Here's how the part is built. I have some questions about the finished solid (model axes, mm). A direction names the side the tool comes from. Coordinates: 2 decimals unless noted, no trailing zeros. Write each loop counter-clockwise with the first axis right and the second up, starting at its lowest first coordinate (ties: lowest second). Pieces come first, ordered by that corner, then holes. Notation, with made-up numbers: M -30.5,-10 L -2.5,-10 A13 ccw -2.5,-6 Z; hole C -31.75,19 d10. An arc over 180 degrees is marked long. Use a Markdown table: item, result.
```python
from build123d import *

# Parameters (mm, degrees)
BOSS_EXTRUDE2_DEPTH      = 3.175
SKETCH4_R                = 38.1
CUT_EXTRUDE3_DEPTH       = 92.247975457
CUT_EXTRUDE6_DEPTH       = 92.247975457
BOSS_EXTRUDE3_DEPTH      = 3.175
SKETCH12_R               = 1.143
CUT_EXTRUDE9_DEPTH       = 97.166400707
SKETCH14_R               = 3.175
CUT_EXTRUDE11_DEPTH      = 103.378
CUT_EXTRUDE11_DEPTH_BACK = 116.832157669
SKETCH15_R               = 1.651
CUT_EXTRUDE12_DEPTH      = 75.692
SKETCH17_R               = 1.651
CUT_EXTRUDE14_DEPTH      = 97.79
SKETCH18_R               = 12.192
CUT_EXTRUDE15_DEPTH      = 35.56


with BuildPart() as part:
    # Sketch1 → Boss-Extrude2 (new body)
    with BuildSketch(Plane.XY):
        with BuildLine():
            Line((-60.107370596, 33.02), (-55.027370596, 33.02))
            Line((-55.027370596, 33.02), (-55.027370596, -33.02))
            Line((-55.027370596, -33.02), (-60.107370596, -33.02))
            ThreePointArc((-60.107370596, -33.02), (0, -68.58), (60.107370596, -33.02))
            Line((60.107370596, -33.02), (55.027370596, -33.02))
            Line((55.027370596, -33.02), (55.027370596, 33.02))
            Line((55.027370596, 33.02), (60.107370596, 33.02))
            ThreePointArc((60.107370596, 33.02), (0, 68.58), (-60.107370596, 33.02))
        make_face()
    extrude(amount=BOSS_EXTRUDE2_DEPTH)

    # Sketch4 → Cut-Extrude3 (cut, through all)
    with BuildSketch(Plane(origin=(0, 0, 0), x_dir=(-1, 0, 0), z_dir=(0, 0, -1))):
        with Locations((0, -86.312058398)):
            Circle(SKETCH4_R)
    extrude(amount=-CUT_EXTRUDE3_DEPTH, mode=Mode.SUBTRACT)

    # Sketch5 → Cut-Extrude6 (cut, through all)
    with BuildSketch(Plane(origin=(0, 0, 0), x_dir=(-1, 0, 0), z_dir=(0, 0, -1))):
        with BuildLine():
            ThreePointArc((45.008715274, -51.743907365), (46.779291091, -50.148921474), (48.493383054, -48.493383054))
            Line((48.493383054, -48.493383054), (33.244765274, -33.244765274))
            Line((33.244765274, -33.244765274), (15.050661462, -15.479201839))
            ThreePointArc((15.050661462, -15.479201839), (11.453327097, -13.609958514), (12.680560823, -17.473736785))
            Line((12.680560823, -17.473736785), (29.410338797, -36.145530887))
            Line((29.410338797, -36.145530887), (45.008715274, -51.743907365))
        make_face()
        with BuildLine():
            ThreePointArc((-48.493383054, -48.493383054), (-46.779291091, -50.148921474), (-45.008715274, -51.743907365))
            Line((-45.008715274, -51.743907365), (-29.410338797, -36.145530887))
            Line((-29.410338797, -36.145530887), (-12.680560823, -17.473736785))
            ThreePointArc((-12.680560823, -17.473736785), (-11.453327097, -13.609958514), (-15.050661462, -15.479201839))
            Line((-15.050661462, -15.479201839), (-33.244765274, -33.244765274))
            Line((-33.244765274, -33.244765274), (-48.493383054, -48.493383054))
        make_face()
        with BuildLine():
            Line((-29.410338797, 36.145530887), (-45.008715274, 51.743907365))
            ThreePointArc((-45.008715274, 51.743907365), (-46.779291091, 50.148921474), (-48.493383054, 48.493383054))
            Line((-48.493383054, 48.493383054), (-33.244765274, 33.244765274))
            Line((-33.244765274, 33.244765274), (-15.050661462, 15.479201839))
            ThreePointArc((-15.050661462, 15.479201839), (-11.453327097, 13.609958514), (-12.680560823, 17.473736785))
            Line((-12.680560823, 17.473736785), (-29.410338797, 36.145530887))
        make_face()
        with BuildLine():
            Line((33.244765274, 33.244765274), (48.493383054, 48.493383054))
            ThreePointArc((48.493383054, 48.493383054), (46.779291091, 50.148921474), (45.008715274, 51.743907365))
            Line((45.008715274, 51.743907365), (29.410338797, 36.145530887))
            Line((29.410338797, 36.145530887), (12.680560823, 17.473736785))
            ThreePointArc((12.680560823, 17.473736785), (11.453327097, 13.609958514), (15.050661462, 15.479201839))
            Line((15.050661462, 15.479201839), (33.244765274, 33.244765274))
        make_face()
    extrude(amount=-CUT_EXTRUDE6_DEPTH, mode=Mode.SUBTRACT)

    # Sketch9 → Boss-Extrude3 (add)
    with BuildSketch(Plane(origin=(0, 0, 0), x_dir=(-1, 0, 0), z_dir=(0, 0, -1))):
        with BuildLine():
            Line((12.7, 67.39381574), (0, 75))
            Line((0, 75), (-12.7, 67.39381574))
            ThreePointArc((-12.7, 67.39381574), (0, 68.58), (12.7, 67.39381574))
        make_face()
    extrude(amount=-BOSS_EXTRUDE3_DEPTH)

    # Sketch12 → Cut-Extrude9 (cut, through all)
    with BuildSketch(Plane(origin=(0, 0, 0), x_dir=(-1, 0, 0), z_dir=(0, 0, -1))):
        with Locations((6.731, 62.23)):
            Circle(SKETCH12_R)
        with Locations((-6.731, 62.23)):
            Circle(SKETCH12_R)
    extrude(amount=-CUT_EXTRUDE9_DEPTH, mode=Mode.SUBTRACT)

    # Sketch14 → Cut-Extrude11 (cut, two sides)
    with BuildSketch(Plane(origin=(30.092005081, 4.08352975, 15.875), x_dir=(-1, 0, 0), z_dir=(0, 0, -1))) as cut_extrude11_sk:
        with Locations(Location((-13.087994919, 21.31647025, 0), (0, 0, 180))):
            Circle(SKETCH14_R)
        with Locations(Location((73.272005081, 21.31647025, 0), (0, 0, 180))):
            Circle(SKETCH14_R)
        with Locations(Location((30.092005081, 21.31647025, 0), (0, 0, 180))):
            Circle(SKETCH14_R)
        with Locations(Location((73.272005081, -29.48352975, 0), (0, 0, 180))):
            Circle(SKETCH14_R)
        with Locations(Location((30.092005081, -29.48352975, 0), (0, 0, 180))):
            Circle(SKETCH14_R)
        with Locations(Location((-13.087994919, -29.48352975, 0), (0, 0, 180))):
            Circle(SKETCH14_R)
    extrude(amount=CUT_EXTRUDE11_DEPTH, mode=Mode.SUBTRACT)
    extrude(cut_extrude11_sk.sketch, amount=-CUT_EXTRUDE11_DEPTH_BACK, mode=Mode.SUBTRACT)

    # Sketch15 → Cut-Extrude12 (cut)
    with BuildSketch(Plane(origin=(30.092005081, 4.08352975, -25.527), x_dir=(-1, 0, 0), z_dir=(0, 0, -1))):
        with Locations(Location((63.757223581, 17.50647025, 0), (0, 0, 180))):
            Circle(SKETCH15_R)
        with Locations(Location((63.757223581, -25.67352975, 0), (0, 0, 180))):
            Circle(SKETCH15_R)
        with Locations(Location((-3.552776419, -25.67352975, 0), (0, 0, 180))):
            Circle(SKETCH15_R)
        with Locations(Location((-3.552776419, 17.50647025, 0), (0, 0, 180))):
            Circle(SKETCH15_R)
    extrude(amount=-CUT_EXTRUDE12_DEPTH, mode=Mode.SUBTRACT)

    # Sketch17 → Cut-Extrude14 (cut)
    with BuildSketch(Plane(origin=(30.092005081, 4.08352975, -31.75), x_dir=(-1, 0, 0), z_dir=(0, 0, -1))):
        with Locations(Location((4.154396091, -49.728759131, 0), (0, 0, 180))):
            Circle(SKETCH17_R)
        with Locations(Location((56.02961407, -49.728759131, 0), (0, 0, 180))):
            Circle(SKETCH17_R)
        with Locations(Location((4.154396091, 41.38247025, 0), (0, 0, 180))):
            Circle(SKETCH17_R)
        with Locations(Location((56.02961407, 41.38247025, 0), (0, 0, 180))):
            Circle(SKETCH17_R)
    extrude(amount=-CUT_EXTRUDE14_DEPTH, mode=Mode.SUBTRACT)

    # Sketch18 → Cut-Extrude15 (cut)
    with BuildSketch(Plane(origin=(0, 0, 0), x_dir=(-1, 0, 0), z_dir=(0, 0, -1))):
        with Locations((31.75, 0)):
            Circle(SKETCH18_R)
        with Locations(Location((-31.75, 0, 0), (0, 0, 180))):
            Circle(SKETCH18_R)
    extrude(amount=-CUT_EXTRUDE15_DEPTH, mode=Mode.SUBTRACT)


solid = part.part
```
1. Suppose I cut it at C-C on z = 1.1. State how many separate pieces and enclosed holes the cut face has, and give its area (3 significant figures).
Answers follow:
| item | result |
|---|---|
| separate pieces | 1 |
| enclosed holes | 18 |
| area | 10,500 mm2 |
2. Which directions (+Z, -Z, +X, -X, +Y, -Y) give clear straight access to the entire face, cutting with the end or side of a thin tool? Please do faces 1 (the face through (54.767, -41.277, 1.565)), 2 (the face through (21.16, -26.94, 1.57)), 3 (the face through (-55.027, 0, 2)).
Answers follow:
| item | result |
|---|---|
| face 1 | +Z, -Z, +X, -Y |
| face 2 | +Z, -Z |
| face 3 | +Z, -Z, -X |
3. We'd pull the mould along X, two halves only. Please class faces 4 (the face through (6.26, 71.25, 1.57)), 5 (the face through (-6.439, 71.144, 1.565)), 6 (the face through (-41, 41, 2)), 7 (the face through (40.01, -25.54, 1.61)): +X half, -X half, draft (parallel to the pull), parting line (faces both ways), or undercut.
Answers follow:
| item | result |
|---|---|
| face 4 | +X half |
| face 5 | -X half |
| face 6 | undercut |
| face 7 | undercut |
4. I need wall thicknesses on probe 1 along X at (y, z) = (42, 0.3); probe 2 along X at (y, z) = (43.5, 1.1); probe 3 along Y at (x, z) = (36, 2.4). Which ranges of each line are inside material? Lowest first, please.
Answers follow:
| item | result |
|---|---|
| probe 1 | x = -54.21 to -42, -35.26 to 35.26, 42 to 54.21 |
| probe 2 | x = -53.02 to -43.5, -36.76 to 36.76, 43.5 to 53.02 |
| probe 3 | y = -58.37 to -42.74, -36 to -11.43, 11.43 to 36, 42.74 to 58.37 |
5. Will these pins go through, and if not, where does the flat tip stop? pin 1 Ø1.5 at (y, z) = (-44.5, 2.5) entering from +X; pin 2 Ø10 at (x, y) = (43.18, 25.4) entering from -Z; pin 3 Ø1.6 at (x, z) = (57, 2) entering from +Y; pin 4 Ø1 at (y, z) = (16.5, 1) entering from +X.
Answers follow:
| item | result |
|---|---|
| pin 1 | stops at x = 52.81 |
| pin 2 | stops at z = 0 |
| pin 3 | stops at y = 39.3 |
| pin 4 | stops at x = 55.03 |
6. Suppose I cut it at A-A on y = 0. Write out the boundary of the cut face in (x, z) (3 decimals), and give its area (3 significant figures).
Answers follow:
| item | result |
|---|---|
| outline | M -55.027,0 L -43.942,0 L -43.942,3.175 L -55.027,3.175 Z; M -19.558,0 L 19.558,0 L 19.558,3.175 L -19.558,3.175 Z; M 43.942,0 L 55.027,0 L 55.027,3.175 L 43.942,3.175 Z |
| area | 195 mm2 |
7. Suppose I cut it at B-B on x = -18. Write out the boundary of the cut face in (y, z) (3 decimals).
Answers follow:
| item | result |
|---|---|
| outline | M -52.732,0 L -23.411,0 L -23.411,3.175 L -52.732,3.175 Z; M -18.359,0 L 18.359,0 L 18.359,3.175 L -18.359,3.175 Z; M 23.411,0 L 66.176,0 L 66.176,3.175 L 23.411,3.175 Z |
